Could you check a few things on this model? Use its own coordinates, in mm. Face numbers are marked on the shaded views. A direction names the side the tool comes from. Coordinates: 2 decimals unless noted, no trailing zeros. Loops run counter-clockwise (first coordinate to the right, second up) from the corner with the lowest first, then second, coordinate; pieces in that order, holes last.
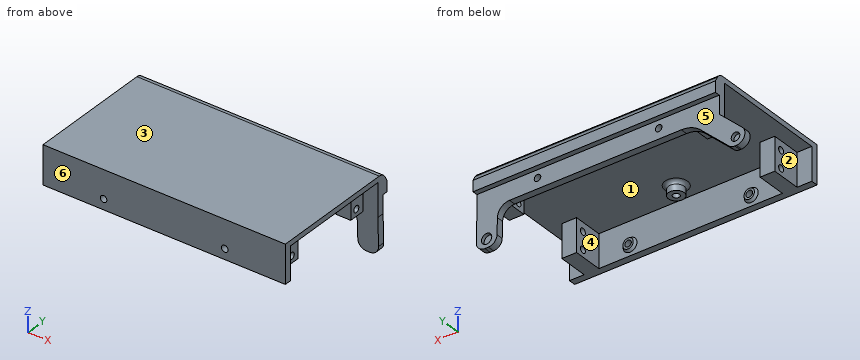
from build123d import *
from OCP.BRepFilletAPI import BRepFilletAPI_MakeChamfer

# Parameters (mm, degrees)
SKETCH1_W               = 140
SKETCH1_H               = 75
BOSS_EXTRUDE1_DEPTH     = 22.2
CUT_EXTRUDE1_DEPTH      = 19.2
CUT_EXTRUDE2_DEPTH      = 147.625679879
CUT_EXTRUDE2_DEPTH_BACK = 147.625679879
SKETCH3_R               = 1.9
CUT_EXTRUDE5_DEPTH      = 103.146169776
CUT_EXTRUDE5_DEPTH_BACK = 103.146169776
SKETCH9_R               = 1.9
BOSS_EXTRUDE6_DEPTH     = 4
FILLET2_R               = 5
BOSS_EXTRUDE10_DEPTH    = 140
FILLET5_R               = 5
SKETCH28_R              = 2.481859786
SKETCH28_R_2            = 2.963166916
CUT_EXTRUDE11_DEPTH     = 2
SKETCH27_R              = 4
SKETCH27_R_2            = 1.9
BOSS_EXTRUDE15_DEPTH    = 1.5
CHAMFER1_SIZE           = 1.5
CHAMFER1_SIZE_2         = 1
SKETCH29_R              = 4.5
SKETCH29_R_2            = 1.9
BOSS_EXTRUDE16_DEPTH    = 5.5
FILLET7_R               = 2


with BuildPart() as part:
    # Sketch1 → Boss-Extrude1 (new body)
    with BuildSketch(Plane.XY):
        Rectangle(SKETCH1_W, SKETCH1_H)
    extrude(amount=BOSS_EXTRUDE1_DEPTH)

    # Sketch2 → Cut-Extrude1 (cut)
    with BuildSketch(Plane(origin=(0, 0, 0), x_dir=(-1, 0, 0), z_dir=(0, 0, -1))):
        Polygon((-61.5, 24), (-53, 24), (-53, 33.5), (53, 33.5), (53, 24), (61.5, 24), (61.5, 33.5), (70, 33.5), (70, 20.2), (70, -20.2), (70, -33.5), (61.5, -33.5), (61.5, -16.4), (53, -16.4), (53, -33.5), (-53, -33.5), (-53, -16.4), (-61.5, -16.4), (-61.5, -33.5), (-70, -33.5), (-70, -20), (-70, 20), (-70, 33.5), (-61.5, 33.5), align=None)
    extrude(amount=-CUT_EXTRUDE1_DEPTH, mode=Mode.SUBTRACT)

    # Sketch3 → Cut-Extrude2 (cut, two sides: drawn at the far end of the back side and taken through both)
    with BuildSketch(Plane.ZY.offset(70).offset(-CUT_EXTRUDE2_DEPTH_BACK)):
        with Locations((14, 28.25)):
            Circle(SKETCH3_R)
        with Locations((4, 28.25)):
            Circle(SKETCH3_R)
        with Locations((4, -21.25)):
            Circle(SKETCH3_R)
        with Locations((14, -21.25)):
            Circle(SKETCH3_R)
    extrude(amount=CUT_EXTRUDE2_DEPTH + CUT_EXTRUDE2_DEPTH_BACK, mode=Mode.SUBTRACT)

    # Sketch9 → Cut-Extrude5 (cut, two sides: drawn at the far end of the back side and taken through both)
    with BuildSketch(Plane(origin=(0, -33.5, 0), x_dir=(1, 0, 0), z_dir=(0, 1, 0)).offset(-CUT_EXTRUDE5_DEPTH_BACK)):
        with Locations(Location((35, -6, 0), (0, 0, 270))):
            Circle(SKETCH9_R)
        with Locations(Location((-35, -6, 0), (0, 0, 90))):
            Circle(SKETCH9_R)
    extrude(amount=CUT_EXTRUDE5_DEPTH + CUT_EXTRUDE5_DEPTH_BACK, mode=Mode.SUBTRACT)

    # Sketch14 → Boss-Extrude6 (add)
    with BuildSketch(Plane(origin=(0, 37.5, 0), x_dir=(1, 0, 0), z_dir=(0, 1, 0))):
        with BuildLine():
            Line((-92.519742911, 21), (-70, 0))
            Line((-70, 0), (-48.085259489, 0))
            ThreePointArc((-48.085259489, 0), (-54.053646754, 1.133133727), (-59.191444218, 4.374842509))
            Line((-59.191444218, 4.374842509), (-77.019742911, 21))
            Line((-77.019742911, 21), (-92.519742911, 21))
        make_face()
        with BuildLine():
            Line((51.164682821, 0), (70, 0))
            Line((70, 0), (70.5, 21))
            Line((70.5, 21), (58.5, 21))
            Line((58.5, 21), (58.162699537, 6.833380554))
            ThreePointArc((58.162699537, 6.833380554), (56.055166635, 1.991690099), (51.164682821, 0))
        make_face()
    extrude(amount=-BOSS_EXTRUDE6_DEPTH)

    # Fillet2
    fillet2_edges = [part.edges().sort_by_distance(p)[0] for p in [
        (-92.519742911, 35.5, -21),
        (-77.019742911, 35.5, -21),
        (58.5, 35.5, -21),
        (70.5, 35.5, -21),
    ]]
    fillet(fillet2_edges, radius=FILLET2_R)

    # Sketch19 → Boss-Extrude10 (add)
    with BuildSketch(Plane.ZY.offset(70)):
        Polygon((10.5, 37.5), (22.2, 37.5), (16.799018003, 40.5), (10.5, 40.5), align=None)
    extrude(amount=-BOSS_EXTRUDE10_DEPTH)

    # Fillet5
    fillet5_edges = [part.edges().sort_by_distance(p)[0] for p in [
        (0, 37.5, 22.2),
    ]]
    fillet(fillet5_edges, radius=FILLET5_R)

    # Sketch28 → Cut-Extrude11 (cut)
    with BuildSketch(Plane(origin=(0, 37.5, 0), x_dir=(1, 0, 0), z_dir=(0, 1, 0))):
        with Locations(Location((-79.386619677, 16, 0), (0, 0, 270))):
            Circle(SKETCH28_R)
        with Locations(Location((64.379251942, 16, 0), (0, 0, 270))):
            Circle(SKETCH28_R_2)
    extrude(amount=-CUT_EXTRUDE11_DEPTH, mode=Mode.SUBTRACT)

    # Sketch27 → Boss-Extrude15 (add)
    # profile 1 of 2: a face of its own
    with BuildSketch(Plane(origin=(0, -33.5, 0), x_dir=(1, 0, 0), z_dir=(0, 1, 0))):
        with Locations(Location((35, -6, 0), (0, 0, 90))):
            Circle(SKETCH27_R)
        with Locations(Location((35, -6, 0), (0, 0, 270))):
            Circle(SKETCH27_R_2, mode=Mode.SUBTRACT)
    # profile 2 of 2: a face of its own
    with BuildSketch(Plane(origin=(0, -33.5, 0), x_dir=(1, 0, 0), z_dir=(0, 1, 0))):
        with Locations(Location((-35, -6, 0), (0, 0, 90))):
            Circle(SKETCH27_R)
        with Locations(Location((-35, -6, 0), (0, 0, 270))):
            Circle(SKETCH27_R_2, mode=Mode.SUBTRACT)
    extrude(amount=BOSS_EXTRUDE15_DEPTH)

    # Chamfer1
    chamfer1_edges_1 = [part.edges().sort_by_distance(p)[0] for p in [
        (35, -32, 10),
    ]]
    chamfer1_side_1 = [part.faces().sort_by_distance(p)[0] for p in [
        (35, -32.02, 10),
    ]]
    chamfer1_edges_2 = [part.edges().sort_by_distance(p)[0] for p in [
        (-35, -32, 10),
    ]]
    chamfer1_side_2 = [part.faces().sort_by_distance(p)[0] for p in [
        (-35, -32.02, 10),
    ]]
    chamfer1 = BRepFilletAPI_MakeChamfer(part.part.solid().wrapped)
    for e in chamfer1_edges_1:
        chamfer1.Add(CHAMFER1_SIZE - 0.0001, CHAMFER1_SIZE_2 - 0.0001, e.wrapped, chamfer1_side_1[0].wrapped)
    for e in chamfer1_edges_2:
        chamfer1.Add(CHAMFER1_SIZE - 0.0001, CHAMFER1_SIZE_2 - 0.0001, e.wrapped, chamfer1_side_2[0].wrapped)
    add(Compound.cast(chamfer1.Shape()), mode=Mode.REPLACE)  # a hair under: the kernel refuses the full size

    # Sketch29 → Boss-Extrude16 (add)
    # profile 1 of 2: a face of its own
    with BuildSketch(Plane(origin=(0, 0, 19.2), x_dir=(-1, 0, 0), z_dir=(0, 0, -1))):
        with Locations((0, 22.5)):
            Circle(SKETCH29_R)
        with Locations((0, 22.5)):
            Circle(SKETCH29_R_2, mode=Mode.SUBTRACT)
    # profile 2 of 2: a face of its own
    with BuildSketch(Plane(origin=(0, 0, 19.2), x_dir=(-1, 0, 0), z_dir=(0, 0, -1))):
        with Locations((0, -22.5)):
            Circle(SKETCH29_R)
        with Locations((0, -22.5)):
            Circle(SKETCH29_R_2, mode=Mode.SUBTRACT)
    extrude(amount=BOSS_EXTRUDE16_DEPTH)

    # Fillet7
    fillet7_edges = [part.edges().sort_by_distance(p)[0] for p in [
        (4.5, 22.5, 19.2),
        (4.5, -22.5, 19.2),
    ]]
    fillet(fillet7_edges, radius=FILLET7_R)


solid = part.part
1) We'd pull the mould along X, two halves only. Please class the marked faces 1, 2 and 3: released by +X, released by -X, zero draft, split by the parting line, or undercut.
2) Imagine slicing it at C-C on y = 3. List the corners of the cut face in (x, z) for me, plus the area to 3 significant figures.
3) Will these pins go through, and if not, where does the flat tip stop? pin 1 (24.5 mm diameter, centred on y = 11, z = 11.5, fed in from -X); pin 2 (2 mm diameter, centred on y = 25, z = 7, fed in from -X); pin 3 (5 mm diameter, centred on x = -65.5, z = -16, fed in from -Y); pin 4 (24.5 mm diameter, centred on y = 5.5, z = 12.5, fed in from +X).
4) Imagine slicing it at A-A on x = 35. State how many separate pieces and enclosed holes the cut face has, plus the area to 3 significant figures.
5) Imagine slicing it at D-D on x = 55.5. List the corners of the cut face in (y, z) for me.
6) If I drill on L1, parallel to Y at x = 0, z = 16; L2, parallel to Y at x = -59, z = 4; L3, parallel to Z at x = 59, y = -21, over which ranges is the centre line in solid material (lowest first)?
7) For the marked faces 4, 5 and 6, which set-ups out of +Z, -Z, +X, -X, +Y, -Y let a thin tool reach every point of the face, with its end or its side?
Solved:
1. face 1: undercut
1. face 2: released by -X
1. face 3: zero draft
2. outline: (-70, 19.2) - (70, 19.2) - (70, 22.2) - (-70, 22.2) - close
2. area: 420 mm2
3. pin 1: stops at x = -70
3. pin 2: stops at x = -61.5
3. pin 3: passes through
3. pin 4: stops at x = 70
4. separate pieces: 3
4. enclosed holes: 0
4. area: 379 mm2
5. outline: (-37.5, 0) - (-16.4, 0) - (-16.4, 19.2) - (24, 19.2) - (24, 0) - (33.5, 0) - (33.5, -1.5) - (37.5, -1.5) - (37.5, 10.5) - (40.5, 10.5) - (40.5, 16.8) - (38.93, 19.63) arc R5 ccw to (34.56, 22.2) - (-37.5, 22.2) - close; hole circle Ø3.8 at (-21.25, 4); hole circle Ø3.8 at (-21.25, 14); hole circle Ø3.8 at (28.25, 4); hole circle Ø3.8 at (28.25, 14)
6. L1: y = -37.5 to -33.5, -27 to -24.4, -20.6 to -18, 18 to 20.6, 24.4 to 27, 33.5 to 40.5
6. L2: y = -37.5 to -23.15, -19.35 to -16.4, 24 to 26.35, 30.15 to 37.5
6. L3: z = 0 to 2.12, 5.88 to 12.12, 15.88 to 22.2
7. face 4: -Z
7. face 5: -Z, +X, -X, +Y
7. face 6: +Z, -Z, +X, -X, -Y
